Check sheet for the drawn part. Datum: minimum x, y, z corner. Units: mm. A direction names the side the tool comes from. Round coordinates to 2 decimals unless told otherwise and drop trailing zeros. Write each loop counter-clockwise with the first axis right and the second up, starting at its lowest first coordinate (ties: lowest second). Pieces come first, ordered by that corner, then holes. Notation, with made-up numbers: M -15,54 L 39,54 A27 cw 39,82 Z; hole C 80.25,75.5 d7. An arc over 180 degrees is marked long. One line per item, written item: value. Start each with the question number.
Item 1: Tool access check on the marked faces 1 and 2. Record the directions out of +Z, -Z, +X, -X, +Y, -Y that give a thin tool (end or side, any length) a straight path to the whole face; none if there is none.
Item 2: Section check C-C, the plane x = 24.5. Record the cut outline in (y, z).
Item 3: Draft check along X on the marked faces 3, 4 and 5. Enter one of: +X half, -X half, draft (parallel to the pull), parting line (faces both ways), or undercut.
Item 4: Gauge pin test, flat ends, axial feed: pin 1 (1.5 mm diameter, centred on x = 3, y = 12.5, fed in from +Z); pin 2 (2.5 mm diameter, centred on x = 12.88, y = 18.68, fed in from +Z); pin 3 (5 mm diameter, centred on x = 14.5, z = 6.5, fed in from +Y). Record the tip position at first contact, or that the pin passes through.
Item 5: Section check A-A, the plane y = 18.25. Record the cut outline in (x, z), then the cut area to 3 significant figures.
Item 6: Thickness scan on probe 1 along Z at (x, y) = (24.75, 22.25); probe 2 along X at (y, z) = (19.5, 8); probe 3 along Y at (x, z) = (19.25, 9.5). Record the ranges inside material, lowest first. Write a range as from..to.
Item 7: Section check D-D, the plane z = 3. State how many separate pieces and enclosed holes the cut face has, then the cut area to 3 significant figures.
Item 8: Section check B-B, the plane x = 19.25. Record the cut outline in (y, z).
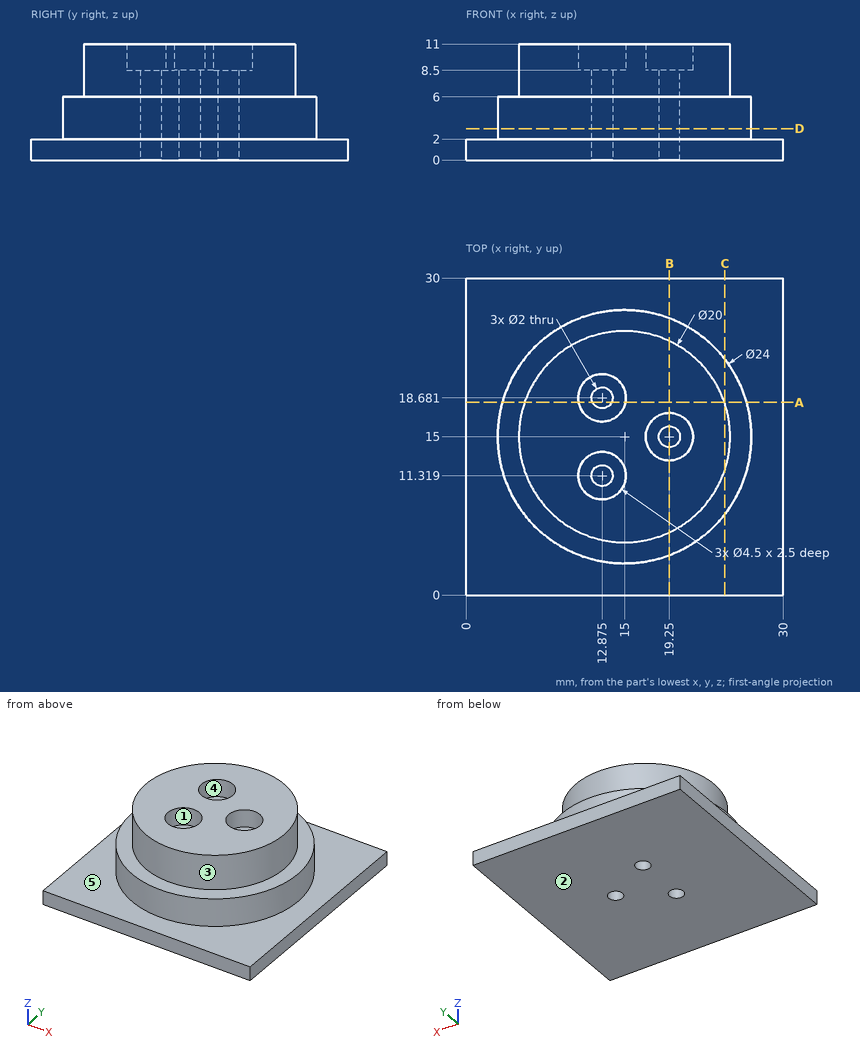
Response values:
1. face 1: +Z
1. face 2: -Z, +X, -X, +Y, -Y
2. outline: M 0,0 L 30,0 L 30,2 L 22.33,2 L 22.33,6 L 18.12,6 L 18.12,11 L 11.88,11 L 11.88,6 L 7.67,6 L 7.67,2 L 0,2 Z
3. face 3: parting line
3. face 4: undercut
3. face 5: draft
4. pin 1: stops at z = 6
4. pin 2: stops at z = 8.5
4. pin 3: stops at y = 27
5. outline: M 0,0 L 11.97,0 L 11.97,8.5 L 10.67,8.5 L 10.67,11 L 5.54,11 L 5.54,6 L 3.45,6 L 3.45,2 L 0,2 Z; M 13.78,0 L 30,0 L 30,2 L 26.55,2 L 26.55,6 L 24.46,6 L 24.46,11 L 15.08,11 L 15.08,8.5 L 13.78,8.5 Z
5. area: 221 mm2
6. probe 1: z = 0..2
6. probe 2: x = 6.07..12.3, 13.45..23.93
6. probe 3: y = 5.95..12.75, 17.25..24.05
7. separate pieces: 1
7. enclosed holes: 3
7. area: 443 mm2
8. outline: M 0,0 L 14,0 L 14,8.5 L 12.75,8.5 L 12.75,11 L 5.95,11 L 5.95,6 L 3.78,6 L 3.78,2 L 0,2 Z; M 16,0 L 30,0 L 30,2 L 26.22,2 L 26.22,6 L 24.05,6 L 24.05,11 L 17.25,11 L 17.25,8.5 L 16,8.5 Z
